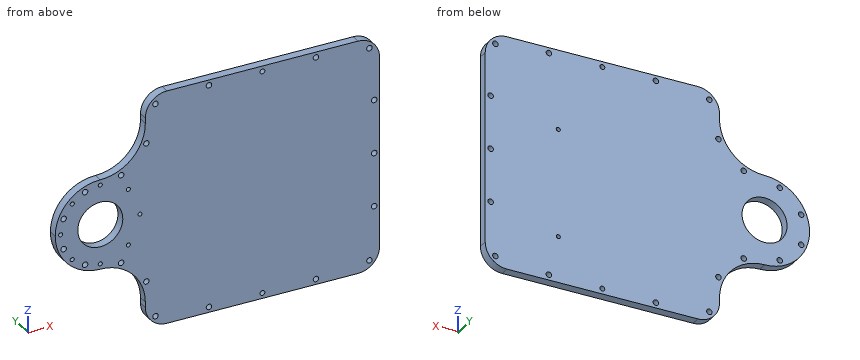
from build123d import *

# Parameters (mm, degrees)
BOSS_EXTRUDE1_DEPTH           = 4
BOSS_EXTRUDE1_DEPTH_BACK      = 1
FILLET1_START                 = -2
FILLET1_DEPTH                 = 7
FILLET1_START_2               = -1
FILLET1_2_DEPTH               = 5
SKETCH39_R                    = 12.5
CUT_EXTRUDE3_DEPTH            = 12.7
TAP_DRILL_FOR_4_40_TAP1_D     = 2.2606
TAP_DRILL_FOR_4_40_TAP1_DEPTH = 2.54
TAP_DRILL_FOR_4_40_TAP1_TIP   = 0.679152758
FILLET2_R                     = 12
SKETCH44_R                    = 1.524
SKETCH44_R_2                  = 1.35
CUT_EXTRUDE4_DEPTH            = 133.193040664
SKETCH47_R                    = 1.1303
CUT_EXTRUDE5_DEPTH            = 2.5


with BuildPart() as part:
    # Sketch1 → Boss-Extrude1 (new, two sides: drawn at the far end of the back side and taken through both)
    with BuildSketch(Plane(origin=(0, 0, 0), x_dir=(1, 0, 0), z_dir=(0, 1, 0)).offset(-BOSS_EXTRUDE1_DEPTH_BACK)):
        Polygon((-65, 25), (-65, 65), (65, 65), (65, -65), (-65, -65), (-65, -25), (-115, -25), (-115, 25), align=None)
    extrude(amount=BOSS_EXTRUDE1_DEPTH + BOSS_EXTRUDE1_DEPTH_BACK)

    # Fillet1: read off the stored shape, not the designer's step
    # Fillet1 outline → Fillet1 (cut)
    with BuildSketch(Plane(origin=(0, 0, 0), x_dir=(1, 0, 0), z_dir=(0, 1, 0)).offset(FILLET1_START)):
        with BuildLine():
            ThreePointArc((-90, -25), (-107.67766953, -17.67766953), (-115, 0))
            Line((-115, 0), (-115, -25))
            Line((-115, -25), (-90, -25))
        make_face()
        with BuildLine():
            ThreePointArc((-115, 0), (-107.67766953, 17.67766953), (-90, 25))
            Line((-90, 25), (-115, 25))
            Line((-115, 25), (-115, 0))
        make_face()
    extrude(amount=FILLET1_DEPTH, mode=Mode.SUBTRACT)

    # Fillet1 2 outline → Fillet1 2 (add)
    with BuildSketch(Plane(origin=(0, 0, 0), x_dir=(1, 0, 0), z_dir=(0, 1, 0)).offset(FILLET1_START_2)):
        with BuildLine():
            Line((-65, 25), (-65, 50))
            ThreePointArc((-65, 50), (-72.32233047, 32.32233047), (-90, 25))
            Line((-90, 25), (-65, 25))
        make_face()
        with BuildLine():
            Line((-65, -25), (-90, -25))
            ThreePointArc((-90, -25), (-72.32233047, -32.32233047), (-65, -50))
            Line((-65, -50), (-65, -25))
        make_face()
    extrude(amount=FILLET1_2_DEPTH)

    # Sketch39 → Cut-Extrude3 (cut)
    with BuildSketch(Plane.XZ.offset(1)):
        with Locations(Location((-90, 0, 0), (0, 0, 270))):
            Circle(SKETCH39_R)
    extrude(amount=-CUT_EXTRUDE3_DEPTH, mode=Mode.SUBTRACT)

    # Tap Drill for #4-40 Tap1
    with Locations(Plane(origin=(0, -1, 0), x_dir=(-1, 0, 0), z_dir=(0, -1, 0))):
        with Locations((90, -22), (74.443650814, -15.556349186), (68, 0), (74.443650814, 15.556349186), (90, 22), (105.556349186, 15.556349186), (112, 0), (105.556349186, -15.556349186)):
            Hole(TAP_DRILL_FOR_4_40_TAP1_D / 2, depth=TAP_DRILL_FOR_4_40_TAP1_DEPTH)
            with Locations((0, 0, -(TAP_DRILL_FOR_4_40_TAP1_DEPTH + TAP_DRILL_FOR_4_40_TAP1_TIP / 2))):  # 118° drill point
                Cone(0, TAP_DRILL_FOR_4_40_TAP1_D / 2, TAP_DRILL_FOR_4_40_TAP1_TIP, mode=Mode.SUBTRACT)

    # Fillet2
    fillet2_edges = [part.edges().sort_by_distance(p)[0] for p in [
        (65, 1.5, -65),
        (65, 1.5, 65),
        (-65, 1.5, 65),
        (-65, 1.5, -65),
    ]]
    fillet(fillet2_edges, radius=FILLET2_R)

    # Sketch44 → Cut-Extrude4 (cut, through all)
    with BuildSketch(Plane.XZ.offset(1)):
        with Locations(Location((-64.419035512, 38.615174316, 0), (0, 0, 270))):
            Circle(SKETCH44_R)
        with Locations(Location((-98.419035512, 20.325349715, 0), (0, 0, 270))):
            Circle(SKETCH44_R)
        with Locations(Location((-110.325349715, 8.419035512, 0), (0, 0, 270))):
            Circle(SKETCH44_R)
        with Locations(Location((-110.325349715, -8.419035512, 0), (0, 0, 270))):
            Circle(SKETCH44_R)
        with Locations(Location((-98.419035512, -20.325349715, 0), (0, 0, 270))):
            Circle(SKETCH44_R)
        with Locations(Location((-64.419035512, -38.615174316, 0), (0, 0, 270))):
            Circle(SKETCH44_R)
        with Locations(Location((-59.363961031, -59.363961031, 0), (0, 0, 270))):
            Circle(SKETCH44_R)
        with Locations(Location((-29.681980515, -62, 0), (0, 0, 270))):
            Circle(SKETCH44_R)
        with Locations(Location((0, -62, 0), (0, 0, 270))):
            Circle(SKETCH44_R_2)
        with Locations(Location((29.681980515, -62, 0), (0, 0, 270))):
            Circle(SKETCH44_R)
        with Locations(Location((59.363961031, -59.363961031, 0), (0, 0, 270))):
            Circle(SKETCH44_R)
        with Locations(Location((62, -29.681980515, 0), (0, 0, 270))):
            Circle(SKETCH44_R)
        with Locations(Location((62, 0, 0), (0, 0, 270))):
            Circle(SKETCH44_R)
        with Locations(Location((62, 29.681980515, 0), (0, 0, 270))):
            Circle(SKETCH44_R)
        with Locations(Location((59.363961031, 59.363961031, 0), (0, 0, 270))):
            Circle(SKETCH44_R)
        with Locations(Location((29.681980515, 62, 0), (0, 0, 270))):
            Circle(SKETCH44_R)
        with Locations(Location((0, 62, 0), (0, 0, 270))):
            Circle(SKETCH44_R_2)
        with Locations(Location((-29.681980515, 62, 0), (0, 0, 270))):
            Circle(SKETCH44_R)
        with Locations(Location((-59.363961031, 59.363961031, 0), (0, 0, 270))):
            Circle(SKETCH44_R)
        with Locations(Location((-78.419035512, -24.507231191, 0), (0, 0, 270))):
            Circle(SKETCH44_R)
        with Locations(Location((-78.419035512, 24.507231191, 0), (0, 0, 270))):
            Circle(SKETCH44_R)
    extrude(amount=-CUT_EXTRUDE4_DEPTH, mode=Mode.SUBTRACT)

    # Sketch47 → Cut-Extrude5 (cut)
    with BuildSketch(Plane(origin=(0, 4, 0), x_dir=(1, 0, 0), z_dir=(0, 1, 0))):
        with Locations(Location((24.46, -20.675, 0), (0, 0, 270))):
            Circle(SKETCH47_R)
        with Locations(Location((24.46, 39.325, 0), (0, 0, 270))):
            Circle(SKETCH47_R)
    extrude(amount=-CUT_EXTRUDE5_DEPTH, mode=Mode.SUBTRACT)


solid = part.part
The listing builds one solid part. Answer for the finished solid, in the listing's coordinates (mm). Coordinates: 2 decimals unless noted, no trailing zeros. Loops run counter-clockwise (first coordinate to the right, second up) from the corner with the lowest first, then second, coordinate; pieces in that order, holes last. Notation, with made-up numbers: (14, -39) -> (56, -39) arc R14 ccw to (56, -12) -> close; hole circle Ø5 at (31, -17). An arc over 180 degrees is marked (long way). Answer in a Markdown table with one row per item. Add a question column.
1. Consider line 1 (Z direction, x = 30, y = 1.4); line 2 (Z direction, x = 1, y = 0.4); line 3 (X direction, y = 0.7, z = -62). Determine where each line is inside the solid, lowest interval first. Write a range as [from, to].
2. The part is cut by section C-C, the plane z = 56. Write down the section's boundary in (x, y).
3. Flat-ended cylindrical pins translate along their axes: P1, Ø4, axis at x = 62, z = 29.68, coming from the +Y side; P2, Ø1, axis at y = 2, z = -5.5, coming from the -X side; P3, Ø1.1, axis at x = 24.5, z = -39.5, coming from the +Y side; P4, Ø2.5, axis at y = 2.5, z = -51, coming from the -X side. Find the tip coordinate at first contact, or state that the pin passes through.
4. The part is cut by section B-B, the plane y = 0. Count the separate pieces of the cut face and the enclosed holes in it, then the cut area to 3 significant figures.
5. The part is cut by section A-A, the plane z = 43. Write down the section's boundary in (x, y).
Answer below:
| question | item | result |
|---|---|---|
| 1 | line 1 | [-65, -63.49], [-60.51, 60.51], [63.49, 65] |
| 1 | line 2 | [-65, -62.91], [-61.09, 61.09], [62.91, 65] |
| 1 | line 3 | [-60.94, -31.21], [-28.16, -1.35], [1.35, 28.16], [31.21, 60.94] |
| 2 | outline | (-64.62, -1) -> (64.62, -1) -> (64.62, 4) -> (-64.62, 4) -> close |
| 3 | P1 | y = 4 |
| 3 | P2 | x = -114.49 |
| 3 | P3 | y = 1.5 |
| 3 | P4 | x = -65 |
| 4 | separate pieces | 1 |
| 4 | enclosed holes | 30 |
| 4 | area | 18,600 mm2 |
| 5 | outline | (-66, -1) -> (65, -1) -> (65, 4) -> (-66, 4) -> close |
